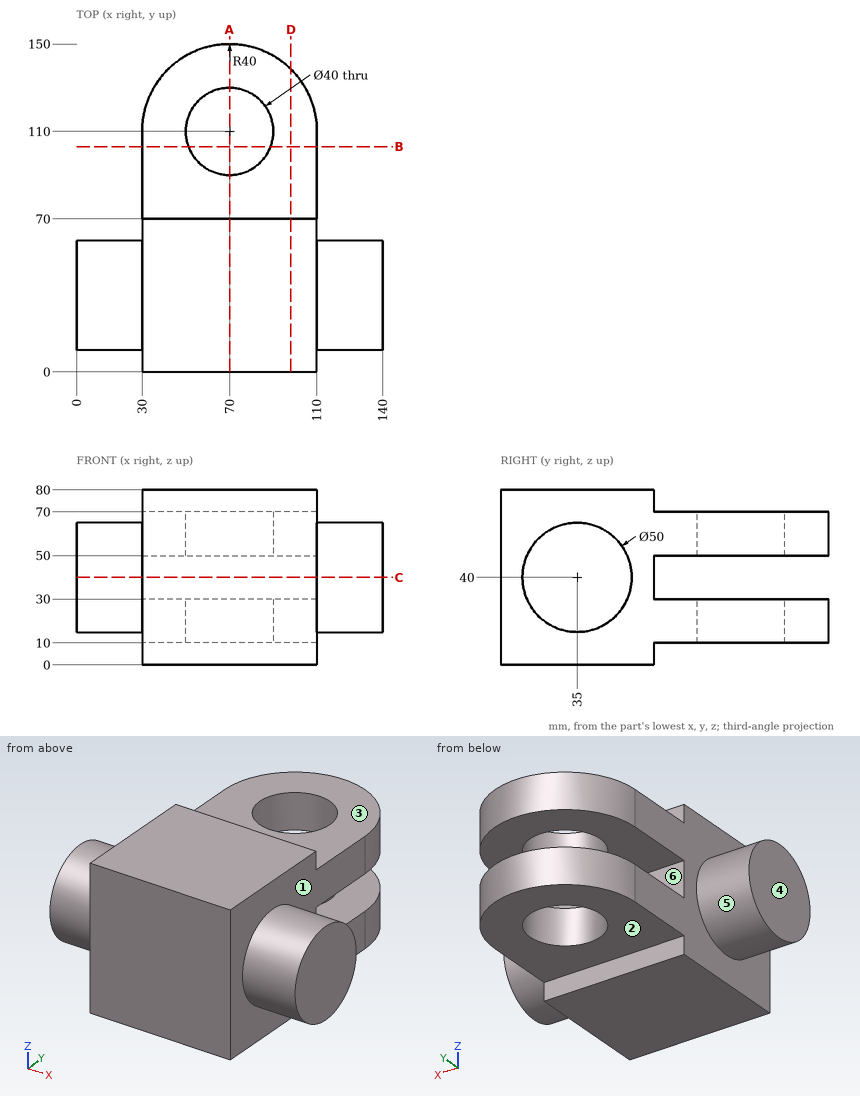
Geometry: see drawing. Coordinates: mm, zero at the bounding-box minimum. A direction names the side the tool comes from. Round coordinates to 2 decimals unless told otherwise and drop trailing zeros. Loops run counter-clockwise (first coordinate to the right, second up) from the corner with the lowest first, then second, coordinate; pieces in that order, holes last. Notation, with made-up numbers: (20, -20) -> (79, -20) arc R20 ccw to (79, 5) -> close; hole circle Ø11 at (54.25, -27.5). An arc over 180 degrees is marked (long way). Use one line per item in the form item = value. Start each with the question number.
Item 1: Section query C-C on z = 40. Return the cut outline in (x, y), then the cut area to 3 significant figures.
Item 2: Section query D-D on x = 98. Return the cut outline in (y, z).
Item 3: Mould query, pull axis Z, two halves, no side actions, for the marked faces 4, 5 and 6. Classes: pulls with the +Z half, pulls with the -Z half, needs draft (parallel to the pull), parting line crosses it, or undercut.
Item 4: Material intervals for L1, parallel to Z at x = 83, y = 134.5; L2, parallel to Y at x = 70, z = 19; L3, parallel to X at y = 91.5, z = 14, sorted ascending. Write a range as from..to.
Item 5: Contact query for flat-ended pins moving along their axis: pin 1 Ø3 at (x, z) = (119, 42) entering from +Y (3 decimals); pin 2 Ø8 at (x, z) = (58.5, 41) entering from +Y; pin 3 Ø5 at (x, z) = (94, 53) entering from +Y. Output: stop coordinate, or through.
Item 6: Set-up query: the marked faces 1, 2 and 3. Return all of +Z, -Z, +X, -X, +Y, -Y with unobstructed straight access to the full face (end or side cutting, diameter ignored); none if empty.
Item 7: Section query A-A on x = 70. Return the cut outline in (y, z).
Item 8: Section query B-B on y = 103. Return the cut outline in (x, z) (3 decimals), then the cut area to 3 significant figures.
Ans:
q1.outline = (0, 10) -> (30, 10) -> (30, 0) -> (110, 0) -> (110, 10) -> (140, 10) -> (140, 60) -> (110, 60) -> (110, 70) -> (30, 70) -> (30, 60) -> (0, 60) -> close
q1.area = 8,600 mm^2
q2.outline = (0, 0) -> (70, 0) -> (70, 10) -> (138.57, 10) -> (138.57, 30) -> (70, 30) -> (70, 50) -> (138.57, 50) -> (138.57, 70) -> (70, 70) -> (70, 80) -> (0, 80) -> close
q3.face_4 = needs draft
q3.face_5 = parting line crosses it
q3.face_6 = undercut
q4.L1 = 10..30, 50..70
q4.L2 = 0..90, 130..150
q4.L3 = 30..62.4, 77.6..110
q5.pin_1 = 59.995
q5.pin_2 = 70
q5.pin_3 = 143.73
q6.face_1 = +X
q6.face_2 = -Z, +X, -X, +Y
q6.face_3 = +Z, +X, -X, +Y
q7.outline = (0, 0) -> (70, 0) -> (70, 10) -> (90, 10) -> (90, 30) -> (70, 30) -> (70, 50) -> (90, 50) -> (90, 70) -> (70, 70) -> (70, 80) -> (0, 80) -> close; (130, 10) -> (150, 10) -> (150, 30) -> (130, 30) -> close; (130, 50) -> (150, 50) -> (150, 70) -> (130, 70) -> close
q8.outline = (30, 10) -> (51.265, 10) -> (51.265, 30) -> (30, 30) -> close; (30, 50) -> (51.265, 50) -> (51.265, 70) -> (30, 70) -> close; (88.735, 10) -> (110, 10) -> (110, 30) -> (88.735, 30) -> close; (88.735, 50) -> (110, 50) -> (110, 70) -> (88.735, 70) -> close
q8.area = 1,700 mm^2
